Autodesk Inventor part; units mm, degrees
ref_plane "YZ Plane" through (0, 0, 0) normal (1, 0, 0) x (0, 1, 0)
ref_plane "XZ Plane" through (0, 0, 0) normal (0, 1, 0) x (-1, 0, 0)
ref_plane "XY Plane" through (0, 0, 0) normal (0, 0, 1) x (1, 0, 0)
sketch "Sketch1" plane through (0, 0, 0) normal (1, 0, 0) x (0, 1, 0)
  arc A0 (0, -19.05) -> (3.175, -22.225) centre (3.175, -19.05) ccw
  arc A1 (19.05, -22.225) -> (22.225, -19.05) centre (19.05, -19.05) ccw
  line L0 (0, -1.4407) -> (0, -19.05)
  line L1 (0.9299, 0.8044) -> (19.515, 19.3894)
  line L2 (22.225, 18.2669) -> (22.225, -19.05)
  line L3 (19.05, -22.225) -> (3.175, -22.225)
  arc A2 (22.225, 18.2669) -> (19.515, 19.3894) centre (20.6375, 18.2669) ccw
  arc A3 (0.9299, 0.8044) -> (0, -1.4407) centre (3.175, -1.4407) ccw
  point P0 (0, -22.225)
  point P1 (22.225, -22.225)
  dimension "d1" = 22.225
  dimension "d6" = 3.175
  dimension "d46" = 1.5875
  dimension "d47" = 3.175
extrude "Extrusion1" add sketch "Sketch1" along normal blind 1.5875
sketch "Sketch2" plane through (1.5875, 0, 0) normal (1, 0, 0) x (0, 0, -1)
  line L0 (22.225, 3.175) -> (22.225, 19.05)
  line L1 (0, 11.1125) -> (4.7625, 11.1125)
  line L2 (4.7625, 11.1125) -> (17.4625, 11.1125)
  line L3 (17.4625, 11.1125) -> (22.225, 11.1125)
  line L4 (4.7625, 11.1125) -> (4.7625, 17.4625)
  line L5 (17.4625, 17.4625) -> (17.4625, 4.7625)
  line L6 (4.7625, 4.7625) -> (4.7625, 11.1125)
  line L7 (4.7625, 17.4625) -> (-17.3369, 17.4625)
  line L8 (-19.3894, 19.515) -> (-0.8044, 0.9299)
  line L9 (-17.3369, 17.4625) -> (-13.9604, 20.8391)
  line L10 (-17.3369, 17.4625) -> (-12.5617, 17.4625) construction
  line L11 (-13.9604, 20.8391) -> (-6.7223, 13.601)
  line L12 (-13.9604, 20.8391) -> (-3.7242, 20.8391) construction
  point P0 (0, 0)
  point P1 (-10.3413, 17.22)
  dimension "d13" = 4.7625
  dimension "d14" = 12.7
  dimension "d15" = 6.35
  dimension "d16" = 12.7
  dimension "d49" = 4.7752
  dimension "d50" = 45
  dimension "d51" = 10.2362
  dimension "d52" = 45
hole "Hole1" at (1.5875, 17.4625, -4.7625) at (1.5875, 4.7625, -4.7625) at (1.5875, 17.22, 10.3413) at (1.5875, 17.4625, -17.4625) at (1.5875, 4.7625, -17.4625) direction (-1, 0, 0) diameter 4.2418 end through all
sketch "Sketch3" plane through (1.5875, 0, 0) normal (1, 0, 0) x (0, 0, -1)
  line L0 (1.4407, 0) -> (19.05, 0)
  line L1 (12.4554, 0) -> (12.4554, 22.225)
  line L2 (19.05, 22.225) -> (-18.2669, 22.225)
  point P0 (0, 0)
split "Split1" [suppressed]
properties part number "sled" material "Polycarbonate, Smoke"
The model under review builds one solid part; all positions refer to its coordinate system, in mm. Give positions to 0.01 mm unless a question says otherwise; leave off trailing zeros. Write each loop counter-clockwise with the first axis right and the second up, starting at its lowest first coordinate (ties: lowest second). Pieces come first, ordered by that corner, then holes.
1. Draft analysis for pull direction Z (two halves, no side actions). For faces 1 (the cylindrical face through (0.783, 2.974, -5.903)), 2 (the cylindrical face through (0.78, 21.32, -21.27)), 3 (the flat face through (0, 13, -6)), state which applies: +Z half, -Z half, draft (parallel to the pull), parting line (faces both ways), or undercut.
2. Add section B-B, the plane z = -16.5. Write out the cut boundary in (x, y) (1 decimal), plus the area to 3 significant figures.
3. Add section C-C, the plane x = 0.85. Count the separate pieces of the cut face and the enclosed holes in it, plus the area to 3 significant figures.
4. Add section A-A, the plane y = 4. Write out the cut boundary in (x, z) (1 decimal), plus the area to 3 significant figures.
5. Add section D-D, the plane y = 18. Write out the cut boundary in (x, z) (1 decimal), plus the area to 3 significant figures.
6. For P1, Ø3, axis at y = 15.5, z = 3.5, coming from the -X side; P2, Ø2.5, axis at y = 17.22, z = 10.34, coming from the -X side, all flat-tipped, find the tip position at first contact; note any pin that passes through.
7. Wall thickness on L1, parallel to Y at x = 1.2, z = -4 (3 decimals); L2, parallel to Z at x = 0.15, y = 17.5 (3 decimals); L3, parallel to Z at x = 0.2, y = 19 (3 decimals): over which ranges is each line inside the solid? List them lowest first.
Worked answers:
1. face 1: undercut
1. face 2: -Z half
1. face 3: draft
2. outline: (0, 0) - (1.6, 0) - (1.6, 2.9) - (0, 2.9) - close; (0, 6.7) - (1.6, 6.7) - (1.6, 15.6) - (0, 15.6) - close; (0, 19.4) - (1.6, 19.4) - (1.6, 22.2) - (0, 22.2) - close
2. area: 23.3 mm2
3. separate pieces: 1
3. enclosed holes: 5
3. area: 660 mm2
4. outline: (0, -22.2) - (1.6, -22.2) - (1.6, -19.4) - (0, -19.4) - close; (0, -15.5) - (1.6, -15.5) - (1.6, -6.7) - (0, -6.7) - close; (0, -2.8) - (1.6, -2.8) - (1.6, 3.9) - (0, 3.9) - close
4. area: 28.9 mm2
5. outline: (0, -22.2) - (1.6, -22.2) - (1.6, -19.5) - (0, -19.5) - close; (0, -15.4) - (1.6, -15.4) - (1.6, -6.8) - (0, -6.8) - close; (0, -2.7) - (1.6, -2.7) - (1.6, 8.4) - (0, 8.4) - close; (0, 12.3) - (1.6, 12.3) - (1.6, 17.9) - (0, 17.9) - close
5. area: 44.4 mm2
6. P1: stops at x = 0
6. P2: passes through
7. L1: y = 0 to 2.783, 6.742 to 15.483, 19.442 to 22.225
7. L2: z = -22.225 to -19.583, -15.342 to -6.883, -2.642 to 8.239, 12.444 to 17.374
7. L3: z = -22.225 to -18.923, -16.002 to -6.223, -3.302 to 9.188, 11.494 to 18.874
